The drawing under review shows one solid part. Ordinate dimensions are in mm from its lowest x, y, z. Coordinates: 2 decimals unless noted, no trailing zeros. Write each loop counter-clockwise with the first axis right and the second up, starting at its lowest first coordinate (ties: lowest second). Pieces come first, ordered by that corner, then holes.
1) We need section B-B on z = 10. Write out the cut boundary in (x, y) (1 decimal).
2) We need section A-A on x = 11. Write out the cut boundary in (y, z) (1 decimal).
3) Mouldability with a two-part tool opening along Z and no side actions: class the marked faces 1, 2 and 3 as pulls with the +Z half, pulls with the -Z half, needs draft (parallel to the pull), parting line crosses it, or undercut.
4) To check wall thickness, follow line 1 along Z through (x, y) = (16, 0.75); line 2 along X through (y, z) = (10, 11.5) (1 decimal); line 3 along X through (y, z) = (4, 17.5) (1 decimal). State the ranges of each line that lie inside material, in increasing order.
5) We need section C-C on x = 24.5. Write out the cut boundary in (y, z) (1 decimal).
6) Insertion check: P1, Ø16.5, axis at x = 15.875, z = 15.875, coming from the -Y side; P2, Ø1.5, axis at y = 5.5, z = 23, coming from the -X side; P3, Ø1.5, axis at x = 12, y = 2.5, coming from the +Z side; P4, Ø1, axis at x = 19.5, y = 8, coming from the -Z side. Each pin has a flat end and moves straight along its axis. Give the tip position at first contact, or say it passes through.
7) We need section D-D on z = 5. Write out the cut boundary in (x, y).
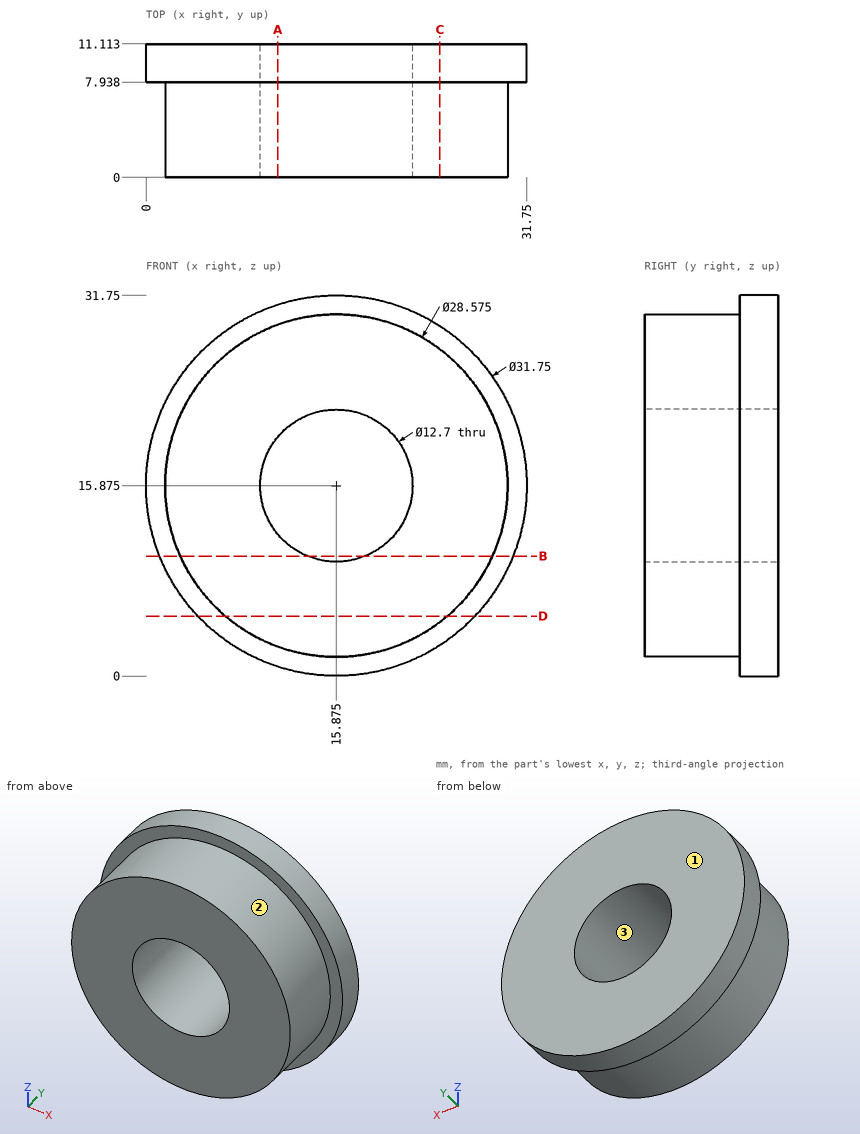
Result:
1. outline: (1.1, 7.9) - (2.9, 7.9) - (2.9, 0) - (13.5, 0) - (13.5, 11.1) - (1.1, 11.1) - close; (18.3, 0) - (28.9, 0) - (28.9, 7.9) - (30.6, 7.9) - (30.6, 11.1) - (18.3, 11.1) - close
2. outline: (0, 2.4) - (7.9, 2.4) - (7.9, 0.8) - (11.1, 0.8) - (11.1, 11.8) - (0, 11.8) - close; (0, 19.9) - (11.1, 19.9) - (11.1, 31) - (7.9, 31) - (7.9, 29.3) - (0, 29.3) - close
3. face 1: needs draft
3. face 2: parting line crosses it
3. face 3: undercut
4. line 1: z = 1.59 to 9.53, 22.22 to 30.16
4. line 2: x = 0.6 to 11.3, 20.5 to 31.1
4. line 3: x = 1.7 to 9.7, 22 to 30.1
5. outline: (0, 4.5) - (7.9, 4.5) - (7.9, 2.5) - (11.1, 2.5) - (11.1, 29.2) - (7.9, 29.2) - (7.9, 27.3) - (0, 27.3) - close
6. P1: stops at y = 0
6. P2: stops at x = 3.09
6. P3: stops at z = 29.82
6. P4: stops at z = 0.31
7. outline: (4.31, 7.94) - (6.61, 7.94) - (6.61, 0) - (25.14, 0) - (25.14, 7.94) - (27.44, 7.94) - (27.44, 11.11) - (4.31, 11.11) - close
